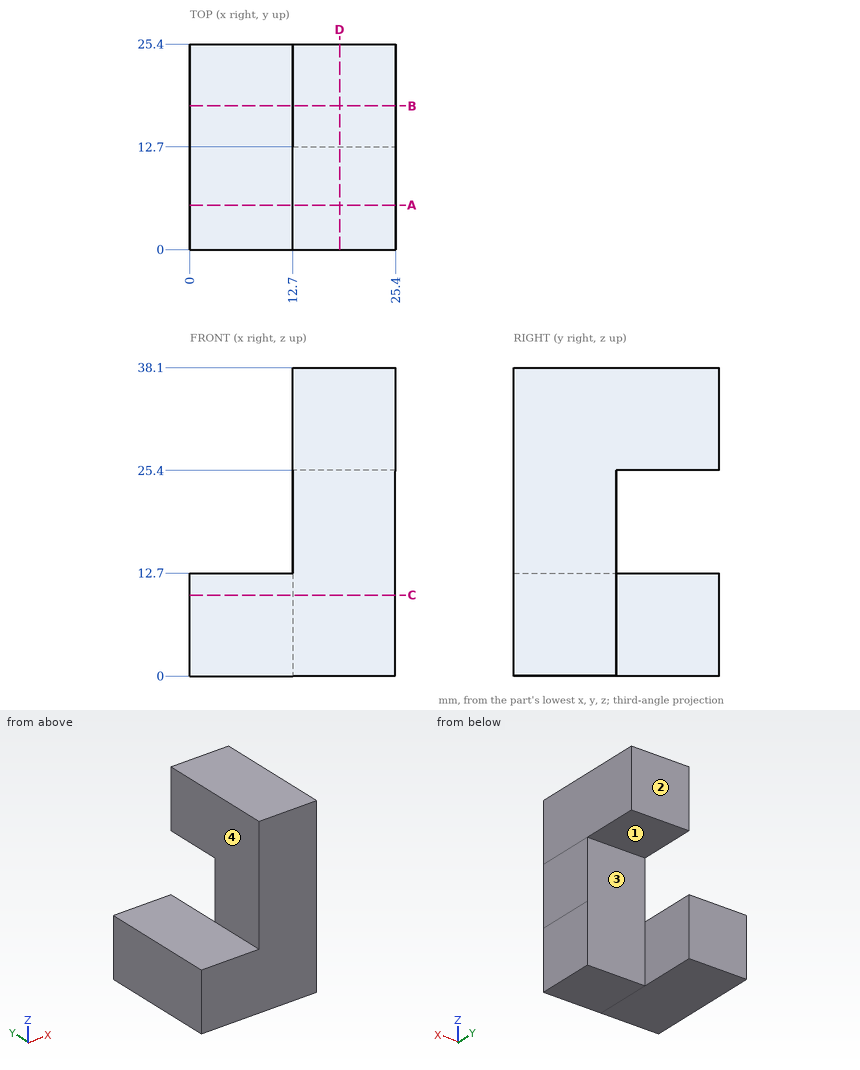
Answer from the drawing. Dimensions are ordinates in mm from the lowest x, y and z of the part. A direction names the side the tool comes from. Coordinates: 2 decimals unless noted, no trailing zeros. Write each loop counter-clockwise with the first axis right and the second up, starting at its lowest first coordinate (ties: lowest second). Pieces come first, ordered by that corner, then holes. Notation, with made-up numbers: (78.5, 81.25) - (131.5, 81.25) arc R31 cw to (131.5, 110.25) - close; hole circle Ø5 at (-13, 65.25). An arc over 180 degrees is marked (long way). One line per question, with ' | ' between items.
Q1. Find section A-A, the plane y = 5.5. Write down the section's boundary in (x, z).
Result set:
outline: (0, 0) - (12.7, 0) - (25.4, 0) - (25.4, 12.7) - (25.4, 25.4) - (25.4, 38.1) - (12.7, 38.1) - (12.7, 12.7) - (0, 12.7) - close
Q2. For the marked faces 1, 2, 3 and 4, determine the directions among +Z, -Z, +X, -X, +Y, -Y from which every point of the face is accessible in a straight line to the end or side of a thin tool.
Result set:
face 1: -Z, +X, -X, +Y | face 2: +Z, -Z, +X, -X, +Y | face 3: -Z, +X, +Y | face 4: +Z, -X, +Y, -Y
Q3. Consider L1, parallel to Z at x = 8.5, y = 17; L2, parallel to X at y = 23.5, z = 30. Determine where each line is inside the solid, lowest interval first. Write a range as [from, to].
Result set:
L1: [0, 12.7] | L2: [12.7, 25.4]
Q4. Each of these flat-tipped pins is pushed along its axis until it touches: P1, Ø7.5, axis at y = 8, z = 25, coming from the -X side; P2, Ø1.5, axis at x = 4, y = 19, coming from the +Z side; P3, Ø4, axis at x = 19.5, z = 12, coming from the +Y side. Where does it stop, or does it pass through?
Result set:
P1: x = 12.7 | P2: z = 12.7 | P3: y = 12.7
Q5. Find section B-B, the plane y = 17.75. Write down the section's boundary in (x, z), plus the area to 3 significant figures.
Result set:
outline: (0, 0) - (12.7, 0) - (12.7, 12.7) - (0, 12.7) - close; (12.7, 25.4) - (25.4, 25.4) - (25.4, 38.1) - (12.7, 38.1) - close | area: 323 mm^2
Q6. Find section C-C, the plane z = 10. Write down the section's boundary in (x, y), plus the area to 3 significant figures.
Result set:
outline: (0, 0) - (25.4, 0) - (25.4, 12.7) - (12.7, 12.7) - (12.7, 25.4) - (0, 25.4) - close | area: 484 mm^2
Q7. Find section D-D, the plane x = 18.5. Write down the section's boundary in (y, z).
Result set:
outline: (0, 0) - (12.7, 0) - (12.7, 25.4) - (25.4, 25.4) - (25.4, 38.1) - (0, 38.1) - close
